Here's how the part is built. I have some questions about the finished solid (model axes, mm). Face numbers are marked on the shaded views. A direction names the side the tool comes from. Coordinates: 2 decimals unless noted, no trailing zeros. Order: outer loops, then holes, each group sorted by start corner. A loop starts at its lowest first (then second) coordinate and runs counter-clockwise, first axis right, second up. Notation, with made-up numbers: (20.25, -18.75) -> (76.25, -18.75) arc R17 cw to (76.25, -12.75) -> close; hole circle Ø4 at (61, 75). An arc over 180 degrees is marked (long way). One line per item, written item: value. Start each with the question number.
```python
from build123d import *

# Parameters (mm, degrees)
SKETCH_1_W           = 52
SKETCH_1_H           = 20
EXTRUDE_4_DEPTH      = 50
SKETCH_11_R          = 21.15
CUT_EXTRUDE_7_DEPTH  = 13
SKETCH_14_R          = 13
CUT_EXTRUDE_9_DEPTH  = 15
CUT_EXTRUDE_13_DEPTH = 35
MM_6_D               = 3.3
MM_6_DEPTH           = 15
MM_6_TIP             = 0.991420021
SKETCH_62_W          = 52
SKETCH_62_H          = 10
CUT_EXTRUDE_14_DEPTH = 97
SKETCH_63_R          = 21.15
CUT_EXTRUDE_15_DEPTH = 2
SKETCH_54_R          = 2
CUT_EXTRUDE_18_DEPTH = 10
SKETCH_76_W          = 52
SKETCH_76_H          = 10
EXTRUDE_7_DEPTH      = 10
F_1_0MM_1_D          = 3.3
F_1_0MM_1_DEPTH      = 15
F_1_0MM_1_TIP        = 0.991420021


with BuildPart() as part:
    # 草图1 → 凸台-拉伸4 (new body)
    with BuildSketch(Plane(origin=(0, 0, 0), x_dir=(1, 0, 0), z_dir=(0, 1, 0))):
        with Locations((26, 10)):
            Rectangle(SKETCH_1_W, SKETCH_1_H)
    extrude(amount=EXTRUDE_4_DEPTH)

    # 草图11 → 切除-拉伸7 (cut)
    with BuildSketch(Plane.XY):
        with Locations((26, 25)):
            Circle(SKETCH_11_R)
    extrude(amount=-CUT_EXTRUDE_7_DEPTH, mode=Mode.SUBTRACT)

    # 草图14 → 切除-拉伸9 (cut)
    with BuildSketch(Plane.XY.offset(-13)):
        with Locations((26, 25)):
            Circle(SKETCH_14_R)
    extrude(amount=-CUT_EXTRUDE_9_DEPTH, mode=Mode.SUBTRACT)

    # 草图56 → 切除-拉伸13 (cut)
    with BuildSketch(Plane(origin=(0, 0, -20), x_dir=(-1, 0, 0), z_dir=(0, 0, -1))):
        Polygon((-38.374368671, 8.125631329), (-52, 8.125631329), (-52, 0), (0, 0), (0, 8.125631329), align=None)
    extrude(amount=-CUT_EXTRUDE_13_DEPTH, mode=Mode.SUBTRACT)

    # 大小mm 暗销孔6
    with Locations(Plane(origin=(3, 8.125631329, -5), x_dir=(-1, 0, 0), z_dir=(0, -1, 0))):
        with Locations((0, 0), (0, 10), (-46, 0), (-46, 10)):
            Hole(MM_6_D / 2, depth=MM_6_DEPTH)
            with Locations((0, 0, -(MM_6_DEPTH + MM_6_TIP / 2))):  # 118° drill point
                Cone(0, MM_6_D / 2, MM_6_TIP, mode=Mode.SUBTRACT)

    # 草图62 → 切除-拉伸14 (cut)
    with BuildSketch(Plane(origin=(0, 50, 0), x_dir=(1, 0, 0), z_dir=(0, 1, 0))):
        with Locations((26, 5)):
            Rectangle(SKETCH_62_W, SKETCH_62_H)
    extrude(amount=-CUT_EXTRUDE_14_DEPTH, mode=Mode.SUBTRACT)

    # 草图63 → 切除-拉伸15 (cut)
    with BuildSketch(Plane.XY.offset(-13)):
        with Locations((26, 25)):
            Circle(SKETCH_63_R)
    extrude(amount=-CUT_EXTRUDE_15_DEPTH, mode=Mode.SUBTRACT)

    # 草图54 → 切除-拉伸18 (cut)
    with BuildSketch(Plane(origin=(0, 0, -20), x_dir=(-1, 0, 0), z_dir=(0, 0, -1))):
        with Locations((-38.374368671, 37.374368671)):
            Circle(SKETCH_54_R)
        with Locations(Location((-13.625631329, 37.374368671, 0), (0, 0, 180))):
            Circle(SKETCH_54_R)
        with Locations((-13.625631329, 12.625631329)):
            Circle(SKETCH_54_R)
        with Locations(Location((-38.374368671, 12.625631329, 0), (0, 0, 180))):
            Circle(SKETCH_54_R)
    extrude(amount=-CUT_EXTRUDE_18_DEPTH, mode=Mode.SUBTRACT)

    # 草图76 → 凸台-拉伸7 (add)
    with BuildSketch(Plane(origin=(0, 50, 0), x_dir=(1, 0, 0), z_dir=(0, 1, 0))):
        with Locations((26, 15)):
            Rectangle(SKETCH_76_W, SKETCH_76_H)
    extrude(amount=EXTRUDE_7_DEPTH)

    # Ø1.0mm 暗销孔1
    with Locations(Plane(origin=(0, 60, 0), x_dir=(1, 0, 0), z_dir=(0, 1, 0))):
        with Locations((3, 15), (49, 15)):
            Hole(F_1_0MM_1_D / 2, depth=F_1_0MM_1_DEPTH)
            with Locations((0, 0, -(F_1_0MM_1_DEPTH + F_1_0MM_1_TIP / 2))):  # 118° drill point
                Cone(0, F_1_0MM_1_D / 2, F_1_0MM_1_TIP, mode=Mode.SUBTRACT)


solid = part.part
```
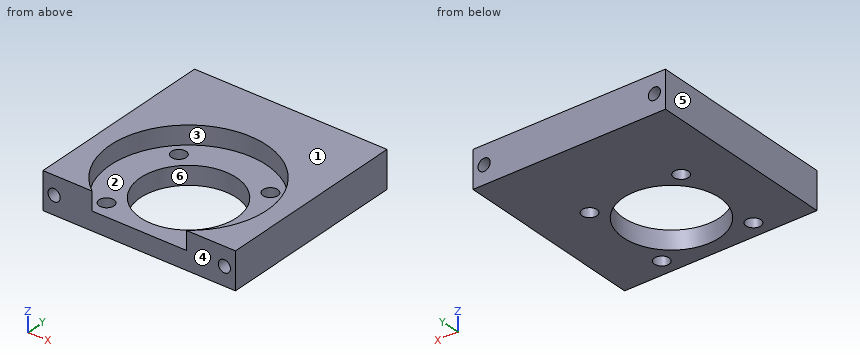
Q1. Imagine slicing it at A-A (y = 25). Write out the boundary of the cut face in (x, z).
Q2. For the marked faces 1 and 2, which set-ups out of +Z, -Z, +X, -X, +Y, -Y let a thin tool reach every point of the face, with its end or its side?
Q3. If we mould it in two halves opening along X, with no side actions, what happens to the marked faces 3, 4, 5 and 6? For each: +X half, -X half, draft (parallel to the pull), parting line (faces both ways), or undercut.
Q4. Imagine slicing it at C-C (y = 47). Write out the boundary of the cut face in (x, z).
Q5. Imagine slicing it at D-D (z = -11.75). Write out the boundary of the cut face in (x, y).
Q6. I need wall thicknesses on line 1 (X direction, y = 52, z = -15); line 2 (Z direction, x = 3, y = 17.75); line 3 (Z direction, x = 45.5, y = 27.5). Which ranges of each line are inside material? Lowest first, please.
Q7. Imagine slicing it at B-B (x = 25). Write out the boundary of the cut face in (y, z).
Q8. For P1, Ø8, axis at x = 35.5, y = 24.5, coming from the -Z side; P2, Ø3.5, axis at x = 13.63, y = 37.37, coming from the -Z side; P3, Ø3, axis at x = 3, z = -15, coming from the -Y side; P4, Ø19, axis at x = 25.5, y = 35, coming from the +Z side, each with a flat end and sliding along its axis, tell me the tip position at first contact or that it passes through.
Completed:
1. outline: (0, -20) -> (13, -20) -> (13, -15) -> (4.85, -15) -> (4.85, -10) -> (0, -10) -> close; (39, -20) -> (52, -20) -> (52, -10) -> (47.15, -10) -> (47.15, -15) -> (39, -15) -> close
2. face 1: +Z, +X, -X, +Y, -Y
2. face 2: +Z
3. face 3: undercut
3. face 4: draft
3. face 5: -X half
3. face 6: undercut
4. outline: (0, -20) -> (52, -20) -> (52, -10) -> (0, -10) -> close; hole circle Ø3.3 at (3, -15); hole circle Ø3.3 at (49, -15)
5. outline: (0, 8.13) -> (13.25, 8.13) arc R21.15 cw (long way) to (38.75, 8.13) -> (52, 8.13) -> (52, 60) -> (0, 60) -> close
6. line 1: x = 0 to 1.35, 4.65 to 47.35, 50.65 to 52
6. line 2: z = -20 to -16.65, -13.35 to -10
6. line 3: z = -20 to -15
7. outline: (8.13, -20) -> (12.04, -20) -> (12.04, -15) -> (8.13, -15) -> close; (37.96, -20) -> (60, -20) -> (60, -10) -> (46.13, -10) -> (46.13, -15) -> (37.96, -15) -> close
8. P1: stops at z = -20
8. P2: passes through
8. P3: stops at y = 23.22
8. P4: stops at z = -15
